Source: CAD feature listing. Evaluate the final solid. Frame: model axes, mm. Give positions to 0.01 mm unless a question says otherwise; leave off trailing zeros. Write each loop counter-clockwise with the first axis right and the second up, starting at its lowest first coordinate (ties: lowest second). Pieces come first, ordered by that corner, then holes. Notation, with made-up numbers: (-9, 86.5) -> (-1, 86.5) arc R23 cw to (-1, 118.5) -> close; hole circle Ø2 at (-38, 51.25). An arc over 180 degrees is marked (long way). Use a Markdown table: item, result. Add a question column.
```python
from build123d import *

# Parameters (mm, degrees)
SKETCH_W      = 25
SKETCH_H      = 69.5
PAD_DEPTH     = 17.5
POCKET_DEPTH  = 4.5
SKETCH003_R   = 2.75
HOLE001_DEPTH = 12
SKETCH004_R   = 2.2
HOLE_DEPTH    = 25.001


with BuildPart() as part:
    # Sketch → Pad (new body, symmetric)
    with BuildSketch(Plane.YZ):
        with Locations((42.5, -44.75)):
            Rectangle(SKETCH_W, SKETCH_H)
    extrude(amount=PAD_DEPTH, both=True)

    # Sketch002 → Pocket (cut)
    with BuildSketch(Plane(origin=(0, 0, -18), x_dir=(0, -1, 0), z_dir=(0, 0, 1))):
        Polygon((-55, -4.25), (-55, 4.25), (-45.046262, 4.25), (-42.592523, 0), (-45.046262, -4.25), align=None)
    extrude(amount=-POCKET_DEPTH, mode=Mode.SUBTRACT)

    # Sketch003 (on Face2 of Pocket) → Hole001 (cut)
    with BuildSketch(Plane(origin=(0, 0, -10), x_dir=(0, -1, 0), z_dir=(0, 0, 1))):
        with Locations((-47.5, 0)):
            Circle(SKETCH003_R)
    extrude(amount=-HOLE001_DEPTH, mode=Mode.SUBTRACT)

    # Sketch004 (on Face6 of Hole001) → Hole (cut, through all)
    with BuildSketch(Plane.ZX.offset(55)):
        with Locations((-72.5, 10.5)):
            Circle(SKETCH004_R)
        with Locations((-56.5, 10.5)):
            Circle(SKETCH004_R)
        with Locations((-72.5, -10.5)):
            Circle(SKETCH004_R)
        with Locations((-56.5, -10.5)):
            Circle(SKETCH004_R)
    extrude(amount=-HOLE_DEPTH, mode=Mode.SUBTRACT)


solid = part.part
```
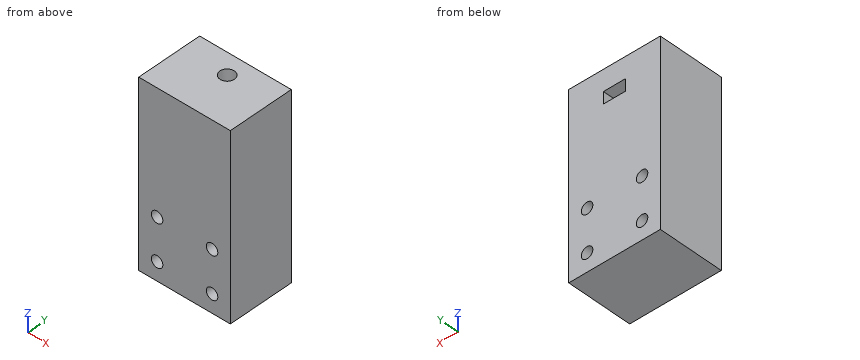
(1) Cut plane D-D on z = -19. Return the cut outline in (x, y), then the cut area to 3 significant figures.
(2) Cut plane C-C on x = -10.5. Return the cut outline in (y, z), then the cut area to 3 significant figures.
(3) Cut plane B-B on y = 47.5. Return the cut outline in (x, z).
(4) Cut plane A-A on z = -72.5. Return the cut outline in (x, y), then the cut area to 3 significant figures.
(5) Material intervals for L1, parallel to X at y = 48, z = -72.5; L2, parallel to X at y = 51, z = -73; L3, parallel to Z at x = -1, y = 53.25, sorted ascending.
Output:
| question | item | result |
|---|---|---|
| 1 | outline | (-17.5, 30) -> (17.5, 30) -> (17.5, 55) -> (4.25, 55) -> (4.25, 45.05) -> (0, 42.59) -> (-4.25, 45.05) -> (-4.25, 55) -> (-17.5, 55) -> close |
| 1 | area | 780 mm^2 |
| 2 | outline | (30, -79.5) -> (55, -79.5) -> (55, -74.7) -> (30, -74.7) -> close; (30, -70.3) -> (55, -70.3) -> (55, -58.7) -> (30, -58.7) -> close; (30, -54.3) -> (55, -54.3) -> (55, -10) -> (30, -10) -> close |
| 2 | area | 1,520 mm^2 |
| 3 | outline | (-17.5, -79.5) -> (17.5, -79.5) -> (17.5, -10) -> (2.75, -10) -> (2.75, -18) -> (4.25, -18) -> (4.25, -22.5) -> (-4.25, -22.5) -> (-4.25, -18) -> (-2.75, -18) -> (-2.75, -10) -> (-17.5, -10) -> close; hole circle Ø4.4 at (-10.5, -72.5); hole circle Ø4.4 at (-10.5, -56.5); hole circle Ø4.4 at (10.5, -72.5); hole circle Ø4.4 at (10.5, -56.5) |
| 4 | outline | (-17.5, 30) -> (-12.7, 30) -> (-12.7, 55) -> (-17.5, 55) -> close; (-8.3, 30) -> (8.3, 30) -> (8.3, 55) -> (-8.3, 55) -> close; (12.7, 30) -> (17.5, 30) -> (17.5, 55) -> (12.7, 55) -> close |
| 4 | area | 655 mm^2 |
| 5 | L1 | -17.5 to -12.7, -8.3 to 8.3, 12.7 to 17.5 |
| 5 | L2 | -17.5 to -12.64, -8.36 to 8.36, 12.64 to 17.5 |
| 5 | L3 | -79.5 to -22.5, -18 to -10 |
